Autodesk Inventor part; units mm, degrees
ref_plane "YZ Plane" through (0, 0, 0) normal (1, 0, 0) x (0, 1, 0)
ref_plane "XZ Plane" through (0, 0, 0) normal (0, 1, 0) x (-1, 0, 0)
ref_plane "XY Plane" through (0, 0, 0) normal (0, 0, 1) x (1, 0, 0)
sketch "Sketch1" plane through (0, 0, 0) normal (0, 0, 1) x (1, 0, 0)
  line L0 (97.5, 9.2765) -> (94.8, 10)
  line L1 (94.8, 10) -> (2.5, 10)
  line L2 (0, 0) -> (100, 0)
  arc A0 (100, 0) -> (97.5, 9.2765) centre (81.5392, 0) ccw
  arc A1 (2.5, 10) -> (0, 0) centre (21.25, 0) ccw
  dimension "d0" = 100
  dimension "d1" = 20
  dimension "d2" = 5.2
  dimension "d3" = 15
  dimension "d4" = 2.5
  dimension "d5" = 2.5
revolve "Body" add sketch "Sketch1" angle 360 about axis through (0, 0, 0) along (1, 0, 0)
sketch "Sketch2" plane through (0, 0, 0) normal (1, 0, 0) x (0, 1, 0)
  circle A0 centre (0, 0) radius 10
  line L0 (0, 10) -> (-1, 10)
  line L1 (0, 10) -> (1, 10)
  line L2 (-1, 10) -> (0, 8.5719)
  line L3 (0, 8.5719) -> (1, 10)
  line L4 (0, -14) -> (0, 14)
  dimension "d6" = 35
  dimension "d7" = 35
  dimension "d8" = 1
extrude "Groove" cut sketch "Sketch2" along normal through all contours L3 L4 A0 | A0 L1 L3 | L4 L2 A0 | A0 L2 L0 picked at (0.5375, 9.5014) picked at (-0.5375, 9.5014)
pattern_circular "Grooves" count 3 over 360 about axis through (-10, 0, 0) along (1, 0, 0) of "Groove"
equation "\"d0\" = NLG"
equation "\"d1\" = NND"
equation "\"d2\" = PHH"
equation "\"d3\" = FAWI"
equation "\"d4\" = KAH"
equation "\"d5\" = KAH"
equation "\"d8\" = 0.05 * NND"
equation "\"NND\" = 20"
equation "\"NLG\" = 100"
equation "\"PHH\" = 5.2"
equation "\"FAWI\" = 15deg"
equation "\"KAH\" = 2.5"
equation "\"d13\" = -KAH"
equation "\"d28\" = KAH"
equation "\"NND1\" = 20.5"
equation "\"KAH1\" = 2"
equation "\"NLG1\" = 98"
properties part number "ISO 8740 - 20 x 100" material "Stainless Steel, Austenitic"
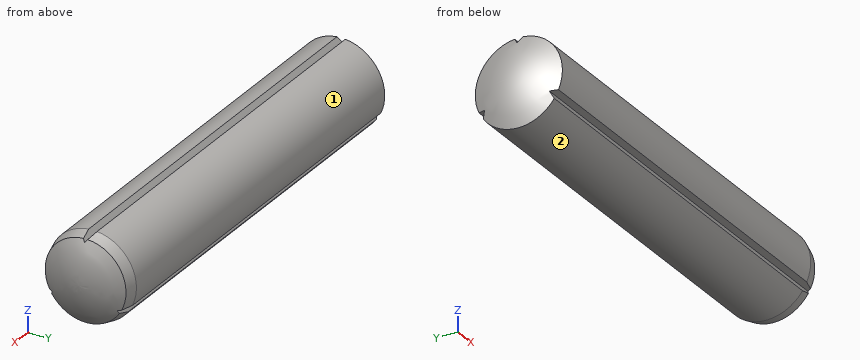
The model under review builds one solid part; all positions refer to its coordinate system, in mm. Face numbers are marked on the shaded views. Coordinates: 2 decimals unless noted, no trailing zeros. Loops run counter-clockwise (first coordinate to the right, second up) from the corner with the lowest first, then second, coordinate; pieces in that order, holes last. Notation, with made-up numbers: (62.5, 10) -> (113.5, 10) arc R19 ccw to (113.5, 28) -> close; hole circle Ø3 at (49.25, -1.75). An arc over 180 degrees is marked (long way). Use a Markdown table: item, result. Add a question column.
1. Clearance check with flat-ended pins moving along their axes: pin 1 Ø1 at (y, z) = (-3, 5) entering from +X; pin 2 Ø3 at (x, y) = (47.5, -3) entering from -Z; pin 3 Ø4 at (x, z) = (20.5, -7.5) entering from +Y; pin 4 Ø12 at (x, y) = (62, -1.5) entering from +Z. State where each tip first meets the part, or that it passes through.
2. Add section A-A on x = 37. Write out the cut boundary in (y, z), plus the area to 3 significant figures.
3. To check wall thickness, follow line 1 (Y direction, x = 39.5, z = 8.75); line 2 (Y direction, x = 42, z = 9); line 3 (Y direction, x = 25, z = -0.5). State the ranges of each line that lie inside material, in increasing order.
4. Draft analysis for pull direction Z (two halves, no side actions). For the marked faces 1 and 2, state which applies: pulls with the +Z half, pulls with the -Z half, needs draft (parallel to the pull), parting line crosses it, or undercut.
Returned:
| question | item | result |
|---|---|---|
| 1 | pin 1 | stops at x = 99.21 |
| 1 | pin 2 | stops at z = -9.89 |
| 1 | pin 3 | stops at y = 8.14 |
| 1 | pin 4 | stops at z = 9.95 |
| 2 | outline | (-9.1, -4.14) -> (-7.42, -4.29) -> (-8.14, -5.81) arc R10 ccw to (8.14, -5.81) -> (7.42, -4.29) -> (9.1, -4.14) arc R10 ccw to (0.97, 9.95) -> (0, 8.57) -> (-0.97, 9.95) arc R10 ccw to start |
| 2 | area | 310 mm² |
| 3 | line 1 | y = -4.84 to -0.12, 0.12 to 4.84 |
| 3 | line 2 | y = -4.36 to -0.3, 0.3 to 4.36 |
| 3 | line 3 | y = -9.99 to 9.99 |
| 4 | face 1 | parting line crosses it |
| 4 | face 2 | pulls with the -Z half |
